Here's how the part is built. I have some questions about the finished solid (model axes, mm). A direction names the side the tool comes from. Coordinates: 2 decimals unless noted, no trailing zeros. Write each loop counter-clockwise with the first axis right and the second up, starting at its lowest first coordinate (ties: lowest second). Pieces come first, ordered by that corner, then holes. Notation, with made-up numbers: (68, 30) -> (94, 30) arc R20 cw to (94, 49) -> close; hole circle Ø7 at (58, 19.5). An arc over 180 degrees is marked (long way). Use a Markdown table: item, result. Add a question column.
Item 1: If we mould it in two halves opening along Z, with no side actions, what happens to faces 1 (the flat face through (-10, 4, -5)), 2 (the cylindrical face through (8.45, 0.51, 3.43)), 3 (the flat face through (10, 17, 5))? For each: pulls with the +Z half, pulls with the -Z half, needs draft (parallel to the pull), parting line crosses it, or undercut.
Item 2: If I drill on line 1 along Z through (x, y) = (9.75, 2); line 2 along X through (y, z) = (1.5, 4.75); line 3 along Z through (x, y) = (5, 20.45), over which ranges is the centre line in solid material (lowest first)? Write a range as from..to.
Item 3: Imagine slicing it at B-B, the plane x = -1. Write out the boundary of the cut face in (y, z), and give its area (3 significant figures).
Item 4: On a 3-axis mill with a long thin cutter (end or side, diameter ignored), from which of +Z, -Z, +X, -X, +Y, -Y can I reach the whole of each face in a straight line? I mean faces 4 (the cylindrical face through (-8.43, 0.51, 3.45)), 5 (the flat face through (-12, 11, 0)), 6 (the cylindrical face through (10.487, 2.479, 4.074)), 7 (the flat face through (8.9, 1, -3.9)), 8 (the flat face through (15.4, 12, 0.5)). Say none if no direction works.
Item 5: Imagine slicing it at A-A, the plane x = -14. Write out the boundary of the cut face in (y, z), and give its area (3 significant figures).
Item 6: Will these pins go through, and if not, where does the flat tip stop? pin 1 Ø4.5 at (x, z) = (5, 0) entering from +Y; pin 2 Ø1 at (x, z) = (9.5, 5) entering from -Y; pin 3 Ø1.5 at (x, z) = (-9, -4.5) entering from -Y.
Item 7: Imagine slicing it at C-C, the plane y = 4.5. Write out the boundary of the cut face in (x, z).
```python
from build123d import *

# Parameters (mm, degrees)
CROQUIS1_W              = 22
CROQUIS1_H              = 12
SALIENTE_EXTRUIR1_DEPTH = 11
CROQUIS3_W              = 10
CROQUIS3_H              = 12
SALIENTE_EXTRUIR2_DEPTH = 2
CROQUIS4_W              = 12
CROQUIS4_H              = 12
SALIENTE_EXTRUIR3_DEPTH = 6
CORTAR_EXTRUIR1_DEPTH   = 2
CROQUIS6_W              = 5
CROQUIS6_H              = 12
SALIENTE_EXTRUIR4_DEPTH = 4
CORTAR_EXTRUIR2_DEPTH   = 4
CROQUIS8_R              = 6
SALIENTE_EXTRUIR5_DEPTH = 4.5
SALIENTE_EXTRUIR6_DEPTH = 4.5
CROQUIS10_W             = 3
CROQUIS10_H             = 3
CORTAR_EXTRUIR3_DEPTH   = 1
REDONDEO1_R             = 1.5
CROQUIS11_W             = 3
CROQUIS11_H             = 3
CORTAR_EXTRUIR4_DEPTH   = 1
REDONDEO3_R             = 1.5
CROQUIS12_R             = 1
CORTAR_EXTRUIR5_DEPTH   = 3
CROQUIS13_R             = 2.5
CORTAR_EXTRUIR6_DEPTH   = 5


with BuildPart() as part:
    # Croquis1 → Saliente-Extruir1 (new body)
    with BuildSketch(Plane(origin=(0, 0, 0), x_dir=(1, 0, 0), z_dir=(0, 1, 0))):
        Rectangle(CROQUIS1_W, CROQUIS1_H)
    extrude(amount=SALIENTE_EXTRUIR1_DEPTH)

    # Croquis3 → Saliente-Extruir2 (add)
    with BuildSketch(Plane(origin=(0, 11, 0), x_dir=(1, 0, 0), z_dir=(0, 1, 0))):
        with Locations((-11, 0)):
            Rectangle(CROQUIS3_W, CROQUIS3_H)
        with Locations((11, 0)):
            Rectangle(CROQUIS3_W, CROQUIS3_H)
    extrude(amount=SALIENTE_EXTRUIR2_DEPTH)

    # Croquis4 → Saliente-Extruir3 (add)
    with BuildSketch(Plane(origin=(0, 11, 0), x_dir=(1, 0, 0), z_dir=(0, 1, 0))):
        Rectangle(CROQUIS4_W, CROQUIS4_H)
    extrude(amount=SALIENTE_EXTRUIR3_DEPTH)

    # Croquis5 → Cortar-Extruir1 (cut)
    with BuildSketch(Plane(origin=(0, 13, 0), x_dir=(1, 0, 0), z_dir=(0, 1, 0))):
        with BuildLine():
            Line((-16, 0), (-16, 0.5))
            Line((-16, 0.5), (-15, 0.5))
            Line((-15, 0.5), (-14.866025404, 0.5))
            ThreePointArc((-14.866025404, 0.5), (-13, 0), (-14.866025404, -0.5))
            Line((-14.866025404, -0.5), (-15, -0.5))
            Line((-15, -0.5), (-15.911665796, -0.5))
            Line((-15.911665796, -0.5), (-16, -0.5))
            Line((-16, -0.5), (-16, 0))
        make_face()
    extrude(amount=-CORTAR_EXTRUIR1_DEPTH, mode=Mode.SUBTRACT)

    # Croquis6 → Saliente-Extruir4 (add)
    with BuildSketch(Plane(origin=(0, 13, 0), x_dir=(1, 0, 0), z_dir=(0, 1, 0))):
        with Locations((-8.5, 0)):
            Rectangle(CROQUIS6_W, CROQUIS6_H)
        with Locations((8.5, 0)):
            Rectangle(CROQUIS6_W, CROQUIS6_H)
    extrude(amount=SALIENTE_EXTRUIR4_DEPTH)

    # Croquis7 → Cortar-Extruir2 (cut)
    with BuildSketch(Plane(origin=(0, 13, 0), x_dir=(1, 0, 0), z_dir=(0, 1, 0))):
        with BuildLine():
            Line((16, 0), (16, 0.5))
            Line((16, 0.5), (14.906951689, 0.5))
            Line((14.906951689, 0.5), (14.866025404, 0.5))
            ThreePointArc((14.866025404, 0.5), (13, 0), (14.866025404, -0.5))
            Line((14.866025404, -0.5), (15, -0.5))
            Line((15, -0.5), (16, -0.5))
            Line((16, -0.5), (16, 0))
        make_face()
    extrude(amount=-CORTAR_EXTRUIR2_DEPTH, mode=Mode.SUBTRACT)

    # Croquis8 → Saliente-Extruir5 (add)
    with BuildSketch(Plane(origin=(0, 17, 0), x_dir=(1, 0, 0), z_dir=(0, 1, 0))):
        with Locations((5, 0)):
            Circle(CROQUIS8_R)
    extrude(amount=SALIENTE_EXTRUIR5_DEPTH)

    # Croquis9 → Saliente-Extruir6 (add)
    with BuildSketch(Plane(origin=(0, 17, 0), x_dir=(1, 0, 0), z_dir=(0, 1, 0))):
        with BuildLine():
            ThreePointArc((-0.454545455, -2.499586743), (-1, 0), (-0.454545455, 2.499586743))
            ThreePointArc((-0.454545455, 2.499586743), (-3, 0), (-0.454545455, -2.499586743))
        make_face()
    extrude(amount=SALIENTE_EXTRUIR6_DEPTH)

    # Croquis10 → Cortar-Extruir3 (cut)
    with BuildSketch(Plane(origin=(0, 0, 0), x_dir=(-1, 0, 0), z_dir=(0, -1, 0))):
        with Locations((9.5, -4.5)):
            Rectangle(CROQUIS10_W, CROQUIS10_H)
    extrude(amount=-CORTAR_EXTRUIR3_DEPTH, mode=Mode.SUBTRACT)

    # Redondeo1
    redondeo1_edges = [part.edges().sort_by_distance(p)[0] for p in [
        (-8, 0.5, 3),
    ]]
    fillet(redondeo1_edges, radius=REDONDEO1_R)

    # Croquis11 → Cortar-Extruir4 (cut)
    with BuildSketch(Plane(origin=(0, 0, 0), x_dir=(-1, 0, 0), z_dir=(0, -1, 0))):
        with Locations((9.5, 4.5)):
            Rectangle(CROQUIS11_W, CROQUIS11_H)
        with Locations((-9.5, -4.5)):
            Rectangle(CROQUIS11_W, CROQUIS11_H)
        with Locations((-9.5, 4.5)):
            Rectangle(CROQUIS11_W, CROQUIS11_H)
    extrude(amount=-CORTAR_EXTRUIR4_DEPTH, mode=Mode.SUBTRACT)

    # Redondeo3
    redondeo3_edges = [part.edges().sort_by_distance(p)[0] for p in [
        (-8, 0.5, -3),
        (8, 0.5, 3),
        (8, 0.5, -3),
    ]]
    fillet(redondeo3_edges, radius=REDONDEO3_R)

    # Croquis12 → Cortar-Extruir5 (cut)
    with BuildSketch(Plane(origin=(0, 1, 0), x_dir=(-1, 0, 0), z_dir=(0, -1, 0))):
        with Locations((9.75, -4.75)):
            Circle(CROQUIS12_R)
        with Locations((9.75, 4.75)):
            Circle(CROQUIS12_R)
        with Locations((-9.75, -4.75)):
            Circle(CROQUIS12_R)
        with Locations((-9.75, 4.75)):
            Circle(CROQUIS12_R)
    extrude(amount=-CORTAR_EXTRUIR5_DEPTH, mode=Mode.SUBTRACT)

    # Croquis13 → Cortar-Extruir6 (cut)
    with BuildSketch(Plane(origin=(0, 21.5, 0), x_dir=(1, 0, 0), z_dir=(0, 1, 0))):
        with Locations((5, 0)):
            Circle(CROQUIS13_R)
    extrude(amount=-CORTAR_EXTRUIR6_DEPTH, mode=Mode.SUBTRACT)


solid = part.part
```
Ans:
| question | item | result |
|---|---|---|
| 1 | face 1 | undercut |
| 1 | face 2 | pulls with the +Z half |
| 1 | face 3 | needs draft |
| 2 | line 1 | z = -6..-5.75, -3.75..3.75, 5.75..6 |
| 2 | line 2 | x = -11..-10.75, -8.75..8.75, 10.75..11 |
| 2 | line 3 | z = -6..-2.5, 2.5..6 |
| 3 | outline | (0, -6) -> (17, -6) -> (17, -2.45) -> (21.5, -2.45) -> (21.5, 2.45) -> (17, 2.45) -> (17, 6) -> (0, 6) -> close |
| 3 | area | 226 mm^2 |
| 4 | face 4 | +Z, -X, -Y |
| 4 | face 5 | +Z, -Z, -X, -Y |
| 4 | face 6 | -Y |
| 4 | face 7 | -Z, +X, -Y |
| 4 | face 8 | +X, +Y, -Y |
| 5 | outline | (11, -6) -> (13, -6) -> (13, -1) -> (11, -1) -> close; (11, 1) -> (13, 1) -> (13, 6) -> (11, 6) -> close |
| 5 | area | 20.0 mm^2 |
| 6 | pin 1 | stops at y = 16.5 |
| 6 | pin 2 | stops at y = 4 |
| 6 | pin 3 | stops at y = 1 |
| 7 | outline | (-11, -6) -> (11, -6) -> (11, 6) -> (-11, 6) -> close |
